from build123d import *

# Parameters (mm, degrees)
SKETCH_1_R      = 1.6
EXTRUDE_1_DEPTH = 3
FILLET_1_R      = 2


with BuildPart() as part:
    # ｽｹｯﾁ1 → ﾎﾞｽ - 押し出し1 (new body)
    with BuildSketch(Plane.XY):
        with BuildLine():
            Line((3, -3.5), (-3, -3.5))
            Line((-3, -3.5), (-3, 3.5))
            ThreePointArc((-3, 3.5), (0, 6.5), (3, 3.5))
            Line((3, 3.5), (3, -3.5))
        make_face()
        with Locations((0, 3.5)):
            Circle(SKETCH_1_R, mode=Mode.SUBTRACT)
    extrude(amount=EXTRUDE_1_DEPTH)

    # ﾌｨﾚｯﾄ1
    fillet_1_edges = [part.edges().sort_by_distance(p)[0] for p in [
        (3, -3.5, 1.5),
        (-3, -3.5, 1.5),
    ]]
    fillet(fillet_1_edges, radius=FILLET_1_R)


solid = part.part
The listing builds one solid part. Answer for the finished solid, in the listing's coordinates (mm). Coordinates: 2 decimals unless noted, no trailing zeros. Write each loop counter-clockwise with the first axis right and the second up, starting at its lowest first coordinate (ties: lowest second). Pieces come first, ordered by that corner, then holes. Notation, with made-up numbers: (30.25, 30) - (68.25, 30) arc R17 ccw to (68.25, 45) - close; hole circle Ø7 at (-9, 34). An arc over 180 degrees is marked (long way). Return JSON: item names as keys, results as strings.
1. Consider line 1 along Y through (x, z) = (0, 2.55); line 2 along Y through (x, z) = (0.5, 0.7); line 3 along Y through (x, z) = (2, 2.2). Determine where each line is inside the solid, lowest interval first.
Final values:
{"line 1": "-3.5 to 1.9, 5.1 to 6.5", "line 2": "-3.5 to 1.98, 5.02 to 6.46", "line 3": "-3.23 to 5.74"}
2. The part is cut by section D-D on y = -2. Determine the outline of the cut face in (x, z).
Final values:
{"outline": "(-2.94, 0) - (2.94, 0) - (2.94, 3) - (-2.94, 3) - close"}
3. For a pull along Y with two mould halves and no side action, classify faces 1 (the face through (1.526, 3.981, 1.479)), 2 (the face through (3, 1, 1)), 3 (the face through (0, -3.5, 1)) as +Y half, -Y half, draft (parallel to the pull), parting line (faces both ways), or undercut.
Final values:
{"face 1": "undercut", "face 2": "draft", "face 3": "-Y half"}
4. The part is cut by section A-A on z = 1.75. Determine the outline of the cut face in (x, y), then the cut area to 3 significant figures.
Final values:
{"outline": "(-3, -1.5) arc R2 ccw to (-1, -3.5) - (1, -3.5) arc R2 ccw to (3, -1.5) - (3, 3.5) arc R3 ccw to (-3, 3.5) - close; hole circle Ø3.2 at (0, 3.5)", "area": "46.4 mm^2"}
5. This flat-tipped pin is pushed along its axis until it touches: pin 1 Ø1 at (x, z) = (-2.5, 2.5) entering from -Y. Where does it stop, or does it pass through?
Final values:
{"pin 1": "y = -3.23"}
6. The part is cut by section C-C on y = 2.25. Determine the outline of the cut face in (x, z), then the cut area to 3 significant figures.
Final values:
{"outline": "(-3, 0) - (-1, 0) - (-1, 3) - (-3, 3) - close; (1, 0) - (3, 0) - (3, 3) - (1, 3) - close", "area": "12.0 mm^2"}
7. The part is cut by section B-B on x = 0. Determine the outline of the cut face in (y, z), then the cut area to 3 significant figures.
Final values:
{"outline": "(-3.5, 0) - (1.9, 0) - (1.9, 3) - (-3.5, 3) - close; (5.1, 0) - (6.5, 0) - (6.5, 3) - (5.1, 3) - close", "area": "20.4 mm^2"}
